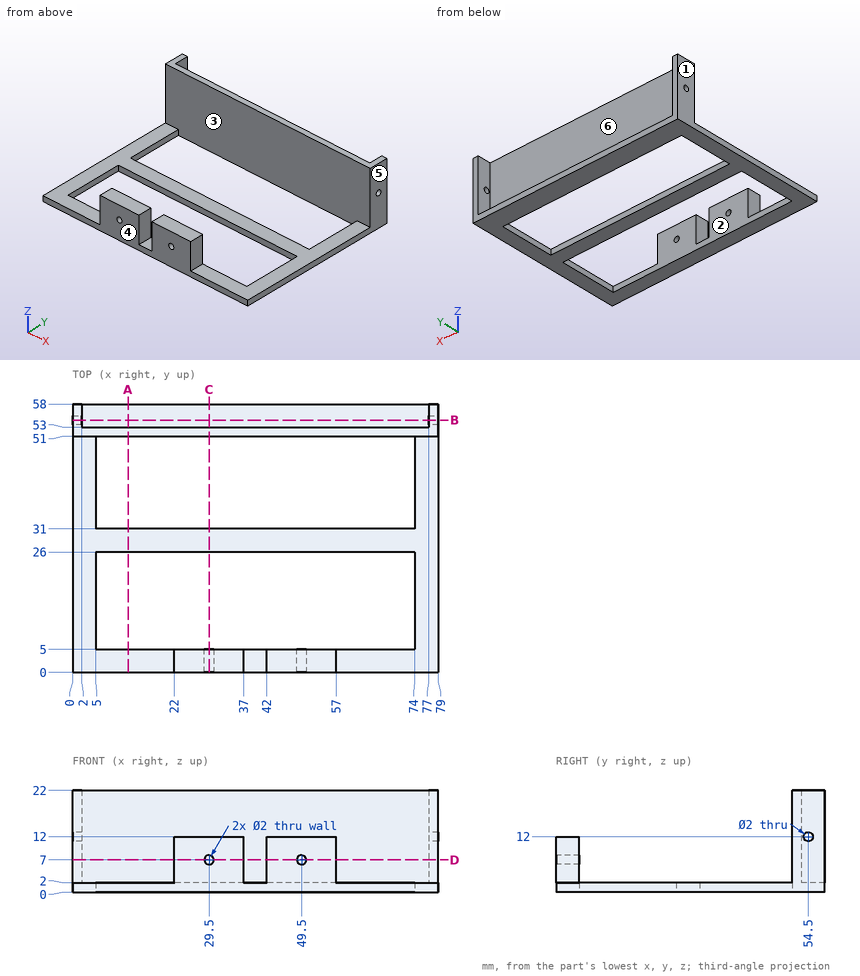
Drawing for the job (mm, zero at the part's lowest x, y, z). A direction names the side the tool comes from. Coordinates: 2 decimals unless noted, no trailing zeros. Write each loop counter-clockwise with the first axis right and the second up, starting at its lowest first coordinate (ties: lowest second). Pieces come first, ordered by that corner, then holes. Notation, with made-up numbers: (16, 9.25) -> (31, 9.25) arc R24 ccw to (31, 22.25) -> close; hole circle Ø10 at (5.5, -9.5). An arc over 180 degrees is marked (long way). One line per item, written item: value. Start each with the question number.
1) Probe probe 1 along X at (y, z) = (39, 1.75); probe 2 along Y at (x, z) = (23.5, 8.5); probe 3 along Y at (x, z) = (1.35, 12). List the from-to ranges inside material, lowest first.
2) Pull direction Y, two halves, no side cores. Call the marked faces 1, 2, 3 and 4: +Y half, -Y half, draft (parallel to the pull), parting line (faces both ways), or undercut.
3) Slice it at D-D on z = 7. Write the cut outline in (x, y).
4) Slice it at A-A on x = 12. Write the cut outline in (y, z), then the cut area to 3 significant figures.
5) Flat gauge pins, fed straight in: pin 1 Ø10 at (x, z) = (64.5, 11) entering from +Y; pin 2 Ø1.5 at (y, z) = (2.5, 6) entering from -X; pin 3 Ø4 at (x, y) = (30, 55.5) entering from +Z. Where does each tip first touch, or does it go through?
6) Slice it at C-C on x = 29.5. Write the cut outline in (y, z).
7) Slice it at B-B on y = 54.5. Write the cut outline in (x, z).
8) Which spindle directions (+Z, -Z, +X, -X, +Y, -Y) get a long thin tool onto all of the face, cutting with end or side? Do the marked faces 5 and 6. Say none if no direction does.
Answers follow:
1. probe 1: 0 to 5, 74 to 79
1. probe 2: 0 to 5, 51 to 53
1. probe 3: 51 to 53.5, 55.5 to 58
2. face 1: draft
2. face 2: undercut
2. face 3: undercut
2. face 4: -Y half
3. outline: (0, 51) -> (79, 51) -> (79, 58) -> (77, 58) -> (77, 53) -> (2, 53) -> (2, 58) -> (0, 58) -> close; (22, 0) -> (28.5, 0) -> (28.5, 5) -> (22, 5) -> close; (30.5, 0) -> (37, 0) -> (37, 5) -> (30.5, 5) -> close; (42, 0) -> (48.5, 0) -> (48.5, 5) -> (42, 5) -> close; (50.5, 0) -> (57, 0) -> (57, 5) -> (50.5, 5) -> close
4. outline: (0, 0) -> (5, 0) -> (5, 2) -> (0, 2) -> close; (26, 0) -> (31, 0) -> (31, 2) -> (26, 2) -> close; (51, 0) -> (58, 0) -> (58, 2) -> (53, 2) -> (53, 22) -> (51, 22) -> close
4. area: 74.0 mm2
5. pin 1: y = 53
5. pin 2: x = 22
5. pin 3: z = 2
6. outline: (0, 0) -> (5, 0) -> (5, 6) -> (0, 6) -> close; (0, 8) -> (5, 8) -> (5, 12) -> (0, 12) -> close; (26, 0) -> (31, 0) -> (31, 2) -> (26, 2) -> close; (51, 0) -> (58, 0) -> (58, 2) -> (53, 2) -> (53, 22) -> (51, 22) -> close
7. outline: (0, 0) -> (79, 0) -> (79, 11) -> (77, 11) -> (77, 2) -> (2, 2) -> (2, 11) -> (0, 11) -> close; (0, 13) -> (2, 13) -> (2, 22) -> (0, 22) -> close; (77, 13) -> (79, 13) -> (79, 22) -> (77, 22) -> close
8. face 5: +Z, -Z, +X, +Y, -Y
8. face 6: +Z, +Y
